from build123d import *

# Parameters (mm, degrees)
MAIN_PROFILE_SKETCH_R          = 1.1
MAIN_EXTRUSION_DEPTH           = 4
DETAIL_PROFILE_2_SKETCH_R      = 2
DETAIL_EXTRUSION_2_DEPTH       = 2
CROSS_BOLT_CLEARANCE_PROFILE_R = 1.1
CROSS_BOLT_CLEARANCE_DEPTH     = 24


with BuildPart() as part:
    # Main Profile Sketch → Main Extrusion (new body)
    with BuildSketch(Plane(origin=(0, -157, 0), x_dir=(-1, 0, 0), z_dir=(0, -1, 0))):
        with BuildLine():
            Line((44.791651246, -3.4278273), (44.791651246, -9))
            Line((44.791651246, -9), (49.791651246, -9))
            Line((49.791651246, -9), (49.791651246, -10.087120501))
            ThreePointArc((49.791651246, -10.087120501), (68.291651246, 0), (49.791651246, 10.087120501))
            Line((49.791651246, 10.087120501), (49.791651246, 9))
            Line((49.791651246, 9), (44.791651246, 9))
            Line((44.791651246, 9), (44.791651246, 3.4278273))
            ThreePointArc((44.791651246, 3.4278273), (44.46433761, 2.02846054), (44.306660633, 0.6))
            Line((44.306660633, 0.6), (50.27147683, 0.6))
            ThreePointArc((50.27147683, 0.6), (62.341651246, 0), (50.27147683, -0.6))
            Line((50.27147683, -0.6), (44.306660633, -0.6))
            ThreePointArc((44.306660633, -0.6), (44.46433761, -2.02846054), (44.791651246, -3.4278273))
        make_face()
        with Locations(Location((65.291651246, 0, 0), (0, 0, 90))):
            Circle(MAIN_PROFILE_SKETCH_R, mode=Mode.SUBTRACT)
        with Locations(Location((56.291651246, 9, 0), (0, 0, 90))):
            Circle(MAIN_PROFILE_SKETCH_R, mode=Mode.SUBTRACT)
        with Locations(Location((56.291651246, -9, 0), (0, 0, 90))):
            Circle(MAIN_PROFILE_SKETCH_R, mode=Mode.SUBTRACT)
    extrude(amount=MAIN_EXTRUSION_DEPTH)

    # Detail Profile 2 Sketch → Detail Extrusion 2 (add)
    with BuildSketch(Plane(origin=(0, -161, 0), x_dir=(-1, 0, 0), z_dir=(0, -1, 0))):
        with BuildLine():
            Line((44.791651246, -3.4278273), (44.791651246, -9))
            Line((44.791651246, -9), (49.791651246, -9))
            Line((49.791651246, -9), (49.791651246, -10.087120501))
            ThreePointArc((49.791651246, -10.087120501), (68.291651246, 0), (49.791651246, 10.087120501))
            Line((49.791651246, 10.087120501), (49.791651246, 9))
            Line((49.791651246, 9), (44.791651246, 9))
            Line((44.791651246, 9), (44.791651246, 3.4278273))
            ThreePointArc((44.791651246, 3.4278273), (44.46433761, 2.02846054), (44.306660633, 0.6))
            Line((44.306660633, 0.6), (50.27147683, 0.6))
            ThreePointArc((50.27147683, 0.6), (62.341651246, 0), (50.27147683, -0.6))
            Line((50.27147683, -0.6), (44.306660633, -0.6))
            ThreePointArc((44.306660633, -0.6), (44.46433761, -2.02846054), (44.791651246, -3.4278273))
        make_face()
        with Locations(Location((65.291651246, 0, 0), (0, 0, 90))):
            Circle(DETAIL_PROFILE_2_SKETCH_R, mode=Mode.SUBTRACT)
        with Locations(Location((56.291651246, 9, 0), (0, 0, 90))):
            Circle(DETAIL_PROFILE_2_SKETCH_R, mode=Mode.SUBTRACT)
        with Locations(Location((56.291651246, -9, 0), (0, 0, 90))):
            Circle(DETAIL_PROFILE_2_SKETCH_R, mode=Mode.SUBTRACT)
    extrude(amount=DETAIL_EXTRUSION_2_DEPTH)

    # Cross Bolt Clearance profile → Cross Bolt Clearance (cut)
    with BuildSketch(Plane.XY.offset(-12)):
        with Locations(Location((-47.291651246, -160, 0), (0, 0, 180))):
            Circle(CROSS_BOLT_CLEARANCE_PROFILE_R)
    extrude(amount=CROSS_BOLT_CLEARANCE_DEPTH, mode=Mode.SUBTRACT)


solid = part.part
Can you work these out from the model? Positions are in its coordinate system, mm. A direction names the side the tool comes from. Give positions to 0.01 mm unless a question says otherwise; leave off trailing zeros. Loops run counter-clockwise (first coordinate to the right, second up) from the corner with the lowest first, then second, coordinate; pieces in that order, holes last. Notation, with made-up numbers: (40.25, 54.25) -> (62.25, 54.25) arc R31 cw to (62.25, 78.25) -> close; hole circle Ø11 at (-1, 44.5). An arc over 180 degrees is marked (long way). Return JSON: item names as keys, results as strings.
Q1. On a 3-axis mill with a long thin cutter (end or side, diameter ignored), from which of +Z, -Z, +X, -X, +Y, -Y can I reach the whole of each face in a straight line? I mean faces 4 (the face through (-49, -160, -0.6)), 5 (the face through (-53, -163, -6)), 6 (the face through (-49.792, -160, 9.5)), 7 (the face through (-57.2, -161, -8.1)). Say none if no direction works.
Checks:
{"face 4": "+X, +Y, -Y", "face 5": "+Z, -Z, +X, -X, -Y", "face 6": "+Z, +X, +Y, -Y", "face 7": "-Y"}
Q2. I need wall thicknesses on probe 1 along Z at (x, y) = (-56.25, -161.8); probe 2 along X at (y, z) = (-159.15, 4.5); probe 3 along Z at (x, y) = (-47.25, -162.7). Which ranges of each line are inside material? Lowest first, please.
Checks:
{"probe 1": "z = -12 to -11, -7 to -6.05, 6.05 to 7, 11 to 12", "probe 2": "x = -67.42 to -60.34, -52.25 to -47.99, -46.59 to -44.79", "probe 3": "z = -9 to -0.6, 0.6 to 9"}
Q3. We'd pull the mould along Z, two halves only. Please class faces 1 (the face through (-44.792, -160, -6)), 2 (the face through (-62.336, -159.958, -0.258)), 3 (the face through (-46, -160, 9)): released by +Z, released by -Z, zero draft, split by the parting line, or undercut.
Checks:
{"face 1": "zero draft", "face 2": "undercut", "face 3": "released by +Z"}
Q4. For pin 1 Ø2.5 at (x, y) = (-47.29, -160) entering from +Z; pin 2 Ø0.5 at (y, z) = (-160.5, 9.5) entering from +X; pin 3 Ø1 at (y, z) = (-161.5, 1.5) entering from -X, each with a flat end and sliding along its axis, tell me the tip position at first contact or that it passes through.
Checks:
{"pin 1": "stops at z = 9", "pin 2": "stops at x = -49.79", "pin 3": "stops at x = -68.25"}
Q5. I want a section at D-D, the plane z = -8.25. List the corners of the cut face in (x, y) for me, then the cut area to 3 significant figures.
Checks:
{"outline": "(-65.01, -163) -> (-58.15, -163) -> (-58.15, -161) -> (-57.1, -161) -> (-57.1, -157) -> (-65.01, -157) -> close; (-55.49, -161) -> (-54.44, -161) -> (-54.44, -163) -> (-44.79, -163) -> (-44.79, -157) -> (-55.49, -157) -> close; hole circle Ø2.2 at (-47.29, -160)", "area": "104 mm2"}
Q6. I want a section at C-C, the plane y = -159.5. List the corners of the cut face in (x, z) for me.
Checks:
{"outline": "(-50.27, -0.6) arc R6.05 cw (long way) to (-50.27, 0.6) -> (-48.27, 0.6) -> (-48.27, 9) -> (-49.79, 9) -> (-49.79, 10.09) arc R12 ccw (long way) to (-49.79, -10.09) -> (-49.79, -9) -> (-48.27, -9) -> (-48.27, -0.6) -> close; (-46.31, -9) -> (-44.79, -9) -> (-44.79, -3.43) arc R12 ccw to (-44.31, -0.6) -> (-46.31, -0.6) -> close; (-46.31, 0.6) -> (-44.31, 0.6) arc R12 ccw to (-44.79, 3.43) -> (-44.79, 9) -> (-46.31, 9) -> close; hole circle Ø2.2 at (-65.29, 0); hole circle Ø2.2 at (-56.29, -9); hole circle Ø2.2 at (-56.29, 9)"}
Q7. I want a section at A-A, the plane x = -49.5. List the corners of the cut face in (y, z) for me, then the cut area to 3 significant figures.
Checks:
{"outline": "(-163, -9) -> (-157, -9) -> (-157, -0.6) -> (-163, -0.6) -> close; (-163, 0.6) -> (-157, 0.6) -> (-157, 9) -> (-163, 9) -> close", "area": "101 mm2"}
Q8. I want a section at B-B, the plane z = 0. List the corners of the cut face in (x, y) for me.
Checks:
{"outline": "(-68.29, -163) -> (-67.29, -163) -> (-67.29, -161) -> (-66.39, -161) -> (-66.39, -157) -> (-68.29, -157) -> close; (-64.19, -161) -> (-63.29, -161) -> (-63.29, -163) -> (-62.34, -163) -> (-62.34, -157) -> (-64.19, -157) -> close"}
